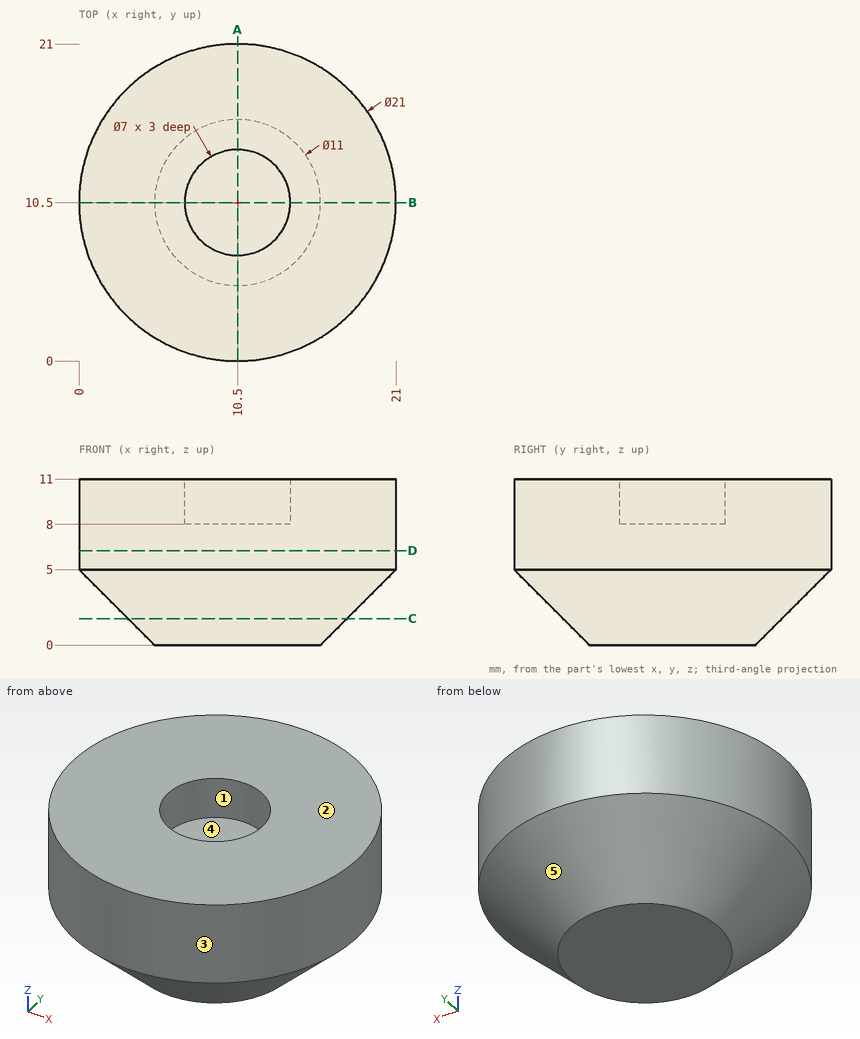
Could you check a few things on this drawing? It's one solid part, dimensions in mm from its lowest x, y, z. A direction names the side the tool comes from. Round coordinates to 2 decimals unless told otherwise and drop trailing zeros. Loops run counter-clockwise (first coordinate to the right, second up) from the corner with the lowest first, then second, coordinate; pieces in that order, holes last. Notation, with made-up numbers: M 87.5,81.25 L 124.5,81.25 A25 cw 124.5,107.25 Z; hole C 85,11.25 d3. An arc over 180 degrees is marked long. Write item = value, one per line. Start each with the question number.
(1) Suppose I cut it at A-A on x = 10.5. Write out the boundary of the cut face in (y, z), plus the area to 3 significant figures.
(2) Suppose I cut it at C-C on z = 1.75. Write out the boundary of the cut face in (x, y), plus the area to 3 significant figures.
(3) I'm going to push flat-ended pins straight in: P1, Ø1.5, axis at x = 9, z = 4, coming from the +Y side; P2, Ø3, axis at y = 5, z = 2.5, coming from the +X side; P3, Ø3, axis at y = 8, z = 2, coming from the +X side. Where does each tip first touch, or does it pass through?
(4) I need wall thicknesses on line 1 along Y through (x, z) = (10.5, 10.2); line 2 along Y through (x, z) = (6.75, 7.75); line 3 along Z through (x, y) = (8, 10.25). Which ranges of each line are inside material? Lowest first, please.
(5) Suppose I cut it at D-D on z = 6.25. Write out the boundary of the cut face in (x, y).
(6) Which directions (+Z, -Z, +X, -X, +Y, -Y) give clear straight access to the entire face, cutting with the end or side of a thin tool? Please do the marked faces 4 and 5.
(7) If we mould it in two halves opening along Y, with no side actions, what happens to the marked faces 1, 2 and 3? For each: released by +Y, released by -Y, zero draft, split by the parting line, or undercut.
Answer block:
q1.outline = M 0,5 L 5,0 L 16,0 L 21,5 L 21,11 L 14,11 L 14,8 L 7,8 L 7,11 L 0,11 Z
q1.area = 185 mm²
q2.outline = C 10.5,10.5 d14.5
q2.area = 165 mm²
q3.P1 = 20.65
q3.P2 = 18.5
q3.P3 = 19.2
q4.line_1 = 0 to 7, 14 to 21
q4.line_2 = 0.69 to 20.31
q4.line_3 = 0 to 8
q5.outline = C 10.5,10.5 d21
q6.face_4 = +Z
q6.face_5 = -Z
q7.face_1 = undercut
q7.face_2 = zero draft
q7.face_3 = split by the parting line
